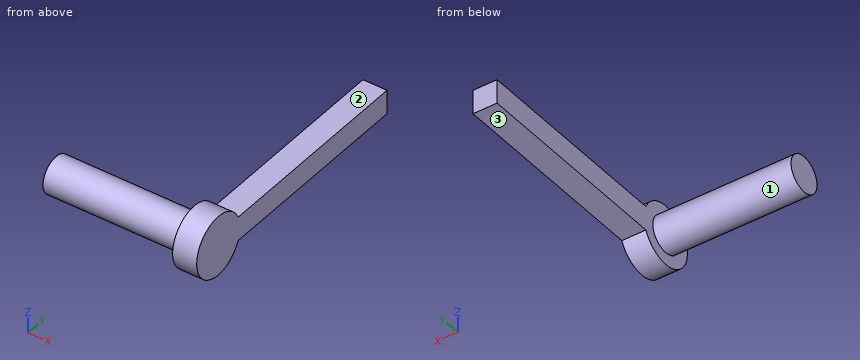
from build123d import *

# Parameters (mm, degrees)
SERVICE_PIN_SHANK_SKETCH_R = 1.5
SERVICE_PIN_SHANK_DEPTH    = 11.5
SERVICE_PIN_HEAD_SKETCH_R  = 2.5
SERVICE_PIN_HEAD_DEPTH     = 2
LOCK_SWITCH_FLAG_SKETCH_W  = 2
LOCK_SWITCH_FLAG_SKETCH_H  = 19.5
LOCK_SWITCH_FLAG_DEPTH     = 2


with BuildPart() as part:
    # Service pin shank sketch → Service pin shank (new body)
    with BuildSketch(Plane(origin=(-12, 0, 0), x_dir=(0, 0, -1), z_dir=(1, 0, 0))):
        with Locations((10.5, -29)):
            Circle(SERVICE_PIN_SHANK_SKETCH_R)
    extrude(amount=SERVICE_PIN_SHANK_DEPTH)

    # Service pin head sketch → Service pin head (add)
    with BuildSketch(Plane(origin=(-0.5, 0, 0), x_dir=(0, 0, -1), z_dir=(1, 0, 0))):
        with Locations((10.5, -29)):
            Circle(SERVICE_PIN_HEAD_SKETCH_R)
    extrude(amount=SERVICE_PIN_HEAD_DEPTH)

    # Lock switch flag sketch → Lock switch flag (add)
    with BuildSketch(Plane.XY.offset(-11.5)):
        with Locations((0.5, -38.75)):
            Rectangle(LOCK_SWITCH_FLAG_SKETCH_W, LOCK_SWITCH_FLAG_SKETCH_H)
    extrude(amount=LOCK_SWITCH_FLAG_DEPTH)


with BuildPart() as body_2:
    # Mirror1: mirrored copy
    add(part.part.mirror(Plane(origin=(0, 0, 0), x_dir=(0, 0, 1), z_dir=(0, -1, 0))))


solid = body_2.part
Part model, mm, in its own coordinate system. Face numbers are marked on the shaded views. A direction names the side the tool comes from. Coordinates: 2 decimals unless noted, no trailing zeros. Loops run counter-clockwise (first coordinate to the right, second up) from the corner with the lowest first, then second, coordinate; pieces in that order, holes last. Notation, with made-up numbers: M 70,-15 L 110,-15 A19 cw 110,-6 Z; hole C 16,44 d11. An arc over 180 degrees is marked long. Use a Markdown table: item, result. Add a question column.
Q1. Probe L1, parallel to X at y = 35.75, z = -9.6; L2, parallel to Y at x = -10.25, z = -11.8; L3, parallel to Y at x = -1.75, z = -10.5. List the from-to ranges inside material, lowest first.
Q2. Cut at C-C (x = -0.75). Write the cut outline in (y, z), and give its area (3 significant figures).
Q3. Which spindle directions (+Z, -Z, +X, -X, +Y, -Y) get a long thin tool onto all of the face, cutting with end or side? Do the marked faces 1, 2 and 3. Say none if no direction does.
Q4. Pin check, flat tips, straight feed: P1, Ø1, axis at y = 42, z = -11, coming from the -X side; P2, Ø0.6, axis at x = 0.5, y = 39, coming from the +Z side; P3, Ø1.5, axis at x = -2.5, y = 34, coming from the -Z side; P4, Ø6, axis at x = -6.5, y = 29.5, coming from the -Z side. Stop position of each tip, or through.
Q5. Cut at B-B (y = 29). Write the cut outline in (x, z), and give its area (3 significant figures).
Q6. Cut at D-D (y = 36.5). Write the cut outline in (x, z).
Q7. Cut at A-A (z = -10.5). Write the cut outline in (x, y).
Worked out:
| question | item | result |
|---|---|---|
| 1 | L1 | x = -0.5 to 1.5 |
| 1 | L2 | y = 28.25 to 29.75 |
| 1 | L3 | y = 27.5 to 30.5 |
| 2 | outline | C 29,-10.5 d3 |
| 2 | area | 7.07 mm2 |
| 3 | face 1 | -X |
| 3 | face 2 | +Z, +X, -X, +Y |
| 3 | face 3 | -Z, +X, -X, +Y |
| 4 | P1 | stops at x = -0.5 |
| 4 | P2 | stops at z = -9.5 |
| 4 | P3 | passes through |
| 4 | P4 | stops at z = -12 |
| 5 | outline | M -12,-12 L -0.5,-12 L -0.5,-13 L 1.5,-13 L 1.5,-8 L -0.5,-8 L -0.5,-9 L -12,-9 Z |
| 5 | area | 44.5 mm2 |
| 6 | outline | M -0.5,-11.5 L 1.5,-11.5 L 1.5,-9.5 L -0.5,-9.5 Z |
| 7 | outline | M -12,27.5 L -0.5,27.5 L -0.5,26.5 L 1.5,26.5 L 1.5,48.5 L -0.5,48.5 L -0.5,30.5 L -12,30.5 Z |
